from build123d import *

# Parameters (mm, degrees)
BOSS_EXTRUDE1_DEPTH            = 7
SKETCH3_R                      = 1.75
CUT_EXTRUDE1_DEPTH             = 124.269646737
CBORE_FOR_M4_SHCS1_D           = 4.5
CBORE_FOR_M4_SHCS1_CBORE_D     = 8
CBORE_FOR_M4_SHCS1_CBORE_DEPTH = 4
FILLET1_R                      = 1
CHAMFER2_SIZE                  = 0.5


with BuildPart() as part:
    # Sketch1 → Boss-Extrude1 (new body)
    with BuildSketch(Plane(origin=(0, 0, 0), x_dir=(1, 0, 0), z_dir=(0, 1, 0))):
        Polygon((43.575468355, 54), (43.575468355, 70), (28.975468355, 70), (28.975468355, 54), (-51.424531645, 54), (-51.424531645, 70), (-66.024531645, 70), (-66.024531645, 54), (-101.224531645, 54), (-101.224531645, -54), (-66.024531645, -54), (-66.024531645, -70), (-51.424531645, -70), (-51.424531645, -54), (28.975468355, -54), (28.975468355, -70), (43.575468355, -70), (43.575468355, -54), (78.775468355, -54), (78.775468355, 54), align=None)
    extrude(amount=BOSS_EXTRUDE1_DEPTH)

    # Sketch3 → Cut-Extrude1 (cut, through all)
    with BuildSketch(Plane.XZ):
        with Locations(Location((33.775468355, 37.5, 0), (0, 0, 270))):
            Circle(SKETCH3_R)
        with Locations(Location((-56.224531645, 37.5, 0), (0, 0, 270))):
            Circle(SKETCH3_R)
        with Locations(Location((73.975468355, 0.7, 0), (0, 0, 270))):
            Circle(SKETCH3_R)
        with Locations(Location((73.975468355, -48.3, 0), (0, 0, 270))):
            Circle(SKETCH3_R)
        with Locations(Location((15.975468355, -48.3, 0), (0, 0, 270))):
            Circle(SKETCH3_R)
        with Locations(Location((15.975468355, 0.7, 0), (0, 0, 270))):
            Circle(SKETCH3_R)
        with Locations(Location((-48.524531645, -4.3, 0), (0, 0, 270))):
            Circle(SKETCH3_R)
        with Locations(Location((-48.524531645, 14.7, 0), (0, 0, 270))):
            Circle(SKETCH3_R)
        with Locations(Location((7.475468355, 14.7, 0), (0, 0, 270))):
            Circle(SKETCH3_R)
        with Locations(Location((7.475468355, -4.3, 0), (0, 0, 270))):
            Circle(SKETCH3_R)
        with Locations(Location((-23.624531645, -13.6, 0), (0, 0, 270))):
            Circle(SKETCH3_R)
        with Locations(Location((-23.624531645, -49.1, 0), (0, 0, 270))):
            Circle(SKETCH3_R)
        with Locations(Location((-74.124531645, -49.1, 0), (0, 0, 270))):
            Circle(SKETCH3_R)
        with Locations(Location((-74.124531645, -13.6, 0), (0, 0, 270))):
            Circle(SKETCH3_R)
        with Locations(Location((-11.574531645, -26, 0), (0, 0, 270))):
            Circle(SKETCH3_R)
        with Locations(Location((3.575468355, -26, 0), (0, 0, 270))):
            Circle(SKETCH3_R)
    extrude(amount=-CUT_EXTRUDE1_DEPTH, mode=Mode.SUBTRACT)

    # CBORE for M4 SHCS1 (through all)
    with Locations(Plane(origin=(0, 7, 0), x_dir=(1, 0, 0), z_dir=(0, 1, 0))):
        with Locations((-58.724531645, 62.5), (36.275468355, 62.5), (36.275468355, -62.5), (-58.724531645, -62.5)):
            CounterBoreHole(CBORE_FOR_M4_SHCS1_D / 2, CBORE_FOR_M4_SHCS1_CBORE_D / 2, CBORE_FOR_M4_SHCS1_CBORE_DEPTH)

    # Fillet1
    fillet1_edges = [part.edges().sort_by_distance(p)[0] for p in [
        (-66.024531645, 3.5, -54),
        (-51.424531645, 3.5, -54),
        (28.975468355, 3.5, -54),
        (43.575468355, 3.5, -54),
        (43.575468355, 3.5, 54),
        (28.975468355, 3.5, 54),
        (-51.424531645, 3.5, 54),
        (-66.024531645, 3.5, 54),
    ]]
    fillet(fillet1_edges, radius=FILLET1_R)

    # Chamfer2
    chamfer2_edges = [part.edges().sort_by_distance(p)[0] for p in [
        (-84.124531645, 0, -54),
        (-66.024531645, 0, -62.5),
        (-66.024531645, 7, 62.5),
        (-84.124531645, 7, 54),
        (-58.724531645, 0, -70),
        (-11.224531645, 7, 54),
        (-11.224531645, 0, 54),
        (-51.424531645, 0, 62.5),
        (28.975468355, 7, 62.5),
        (61.675468355, 0, 54),
        (43.575468355, 0, 62.5),
        (43.575468355, 0, -62.5),
        (61.675468355, 0, -54),
        (-11.224531645, 7, -54),
        (-11.224531645, 0, -54),
        (28.975468355, 0, -62.5),
        (28.975468355, 7, -62.5),
        (-84.124531645, 7, -54),
        (-66.024531645, 7, -62.5),
        (36.275468355, 0, -70),
        (-51.424531645, 0, -62.5),
        (-66.317424864, 0, 54.292893219),
        (-66.317424864, 7, 54.292893219),
        (-51.131638426, 0, 54.292893219),
        (-51.131638426, 7, 54.292893219),
        (28.682575136, 0, 54.292893219),
        (28.682575136, 7, 54.292893219),
        (43.868361574, 0, 54.292893219),
        (43.868361574, 7, 54.292893219),
        (43.868361574, 0, -54.292893219),
        (43.868361574, 7, -54.292893219),
        (28.682575136, 0, -54.292893219),
        (28.682575136, 7, -54.292893219),
        (-66.317424864, 0, -54.292893219),
        (-66.317424864, 7, -54.292893219),
        (-51.131638426, 0, -54.292893219),
        (-51.131638426, 7, -54.292893219),
        (78.775468355, 0, 0),
        (36.275468355, 0, 70),
        (28.975468355, 0, 62.5),
        (-58.724531645, 0, 70),
        (-66.024531645, 0, 62.5),
        (-84.124531645, 0, 54),
        (-101.224531645, 0, 0),
        (-101.224531645, 3.5, -54),
        (-66.024531645, 3.5, -70),
        (-51.424531645, 3.5, -70),
        (-58.724531645, 7, -70),
        (-51.424531645, 7, -62.5),
        (28.975468355, 3.5, -70),
        (43.575468355, 3.5, -70),
        (36.275468355, 7, -70),
        (43.575468355, 7, -62.5),
        (78.775468355, 3.5, -54),
        (61.675468355, 7, -54),
        (78.775468355, 3.5, 54),
        (78.775468355, 7, 0),
        (61.675468355, 7, 54),
        (43.575468355, 3.5, 70),
        (43.575468355, 7, 62.5),
        (28.975468355, 3.5, 70),
        (36.275468355, 7, 70),
        (-51.424531645, 3.5, 70),
        (-51.424531645, 7, 62.5),
        (-66.024531645, 3.5, 70),
        (-58.724531645, 7, 70),
        (-101.224531645, 3.5, 54),
        (-101.224531645, 7, 0),
    ]]
    chamfer(chamfer2_edges, length=CHAMFER2_SIZE)


solid = part.part
Input: part model. Units: mm. Frame: model coordinates. A direction names the side the tool comes from. Coordinates: 2 decimals unless noted, no trailing zeros. Loops run counter-clockwise (first coordinate to the right, second up) from the corner with the lowest first, then second, coordinate; pieces in that order, holes last. Notation, with made-up numbers: (36.25, -23.5) -> (90.25, -23.5) arc R9 ccw to (90.25, -17.5) -> close; hole circle Ø7 at (-21, 77.25). An arc over 180 degrees is marked (long way). Write item = value, one per line. Start each with the question number.
Item 1: Material intervals for line 1 (X direction, y = 4, z = 14.7); line 2 (X direction, y = 4, z = -26); line 3 (Z direction, x = -22.5, y = 5.75), sorted ascending.
Item 2: Cut plane A-A, the plane z = -62.5. Count the separate pieces of the cut face and the enclosed holes in it, plus the area to 3 significant figures.
Item 3: Mould query, pull axis X, two halves, no side actions, for faces 1 (the face through (-59, 3, 70)), 2 (the face through (43.575, 3, -62)), 3 (the face through (-57, 3, -60.8)). Classes: pulls with the +X half, pulls with the -X half, needs draft (parallel to the pull), parting line crosses it, or undercut.
Item 4: Reachability of faces 4 (the face through (28.975, 3, -62)), 5 (the face through (-59.592, 5.028, 66.405)), 6 (the face through (3.65, 3.45, -24.25)) from +Z, -Z, +X, -X, +Y, -Y: full face, straight path, thin tool, end or side. Return the list, or none.
Item 5: First-contact query: P1, Ø2.5, axis at x = -57, z = -61.5, coming from the +Y side; P2, Ø3, axis at x = -77, y = 5, coming from the -Z side. Flat tips, straight axial feed; report the tip coordinate or a pass-through.
Item 6: Cut plane B-B, the plane x = -84. Return loops of the section in (y, z), plus the area to 4 significant figures.
Ans:
q1.line_1 = -101.22 to -50.27, -46.77 to 5.73, 9.23 to 78.78
q1.line_2 = -101.22 to -13.32, -9.82 to 1.83, 5.33 to 78.78
q1.line_3 = -54 to -50.44, -47.76 to -14.94, -12.26 to 54
q2.separate_pieces = 4
q2.enclosed_holes = 0
q2.area = 112 mm²
q3.face_1 = needs draft
q3.face_2 = pulls with the +X half
q3.face_3 = undercut
q4.face_4 = -Z, +Y, -Y
q4.face_5 = +Y
q4.face_6 = +Y, -Y
q5.P1 = 3
q5.P2 = -54
q6.outline = (0, -53.5) -> (0.5, -54) -> (6.5, -54) -> (7, -53.5) -> (7, 53.5) -> (6.5, 54) -> (0.5, 54) -> (0, 53.5) -> close
q6.area = 755.5 mm²
